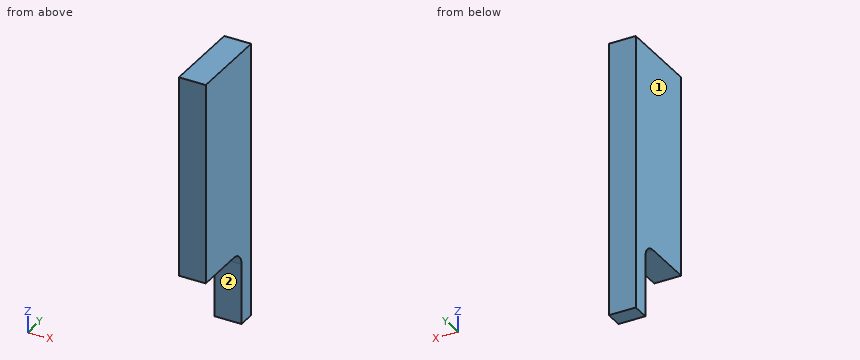
```python
from build123d import *

# Parameters (mm, degrees)
BOSS_EXTRUDE1_DEPTH = 12.7


with BuildPart() as part:
    # Sketch2 → Boss-Extrude1 (new, symmetric)
    with BuildSketch(Plane(origin=(0, 0, 0), x_dir=(0, 0, -1), z_dir=(1, 0, 0))):
        with BuildLine():
            Line((-130, 38.1), (130, 38.1))
            Line((130, 38.1), (130, 21.9))
            Line((130, 21.9), (72.7, 21.9))
            ThreePointArc((72.7, 21.9), (63.719743879, 18.180256121), (60, 9.2))
            Line((60, 9.2), (60, -38.1))
            Line((60, -38.1), (-130, -38.1))
            Line((-130, -38.1), (-130, 38.1))
        make_face()
    extrude(amount=BOSS_EXTRUDE1_DEPTH, both=True)


solid = part.part
```
Input: part model. Units: mm. Frame: model coordinates. Face numbers are marked on the shaded views. A direction names the side the tool comes from. Round coordinates to 2 decimals unless told otherwise and drop trailing zeros. Loops run counter-clockwise (first coordinate to the right, second up) from the corner with the lowest first, then second, coordinate; pieces in that order, holes last.
1) Section query A-A on x = -8.5. Return the cut outline in (y, z), plus the area to 3 significant figures.
Ans:
outline: (-38.1, -60) - (9.2, -60) arc R12.7 cw to (21.9, -72.7) - (21.9, -130) - (38.1, -130) - (38.1, 130) - (-38.1, 130) - close
area: 15,600 mm2
2) Pin query (flat end, axial travel): pin 1 (12.5 mm diameter, centred on x = 2, z = -104.5, fed in from -Y); pin 2 (1.5 mm diameter, centred on x = -7, y = 6, fed in from -Z). Return the tip coordinate at first contact, or that it passes through.
Ans:
pin 1: stops at y = 21.9
pin 2: stops at z = -60
3) Section query C-C on y = 17. Return the cut outline in (x, z), plus the area to 3 significant figures.
Ans:
outline: (-12.7, -62.68) - (12.7, -62.68) - (12.7, 130) - (-12.7, 130) - close
area: 4,890 mm2
4) Material intervals for line 1 (Z direction, x = 8, y = -25); line 2 (Y direction, x = 1.5, z = -93.5); line 3 (Z direction, x = 3.5, y = 19), sorted ascending.
Ans:
line 1: z = -60 to 130
line 2: y = 21.9 to 38.1
line 3: z = -64.62 to 130
5) Set-up query: the marked faces 1 and 2. Return all of +Z, -Z, +X, -X, +Y, -Y with unobstructed straight access to the full face (end or side cutting, diameter ignored); none if empty.
Ans:
face 1: +Z, -Z, -X, +Y, -Y
face 2: -Z, +X, -X, -Y
6) Section query B-B on y = 2.5. Return the cut outline in (x, z).
Ans:
outline: (-12.7, -60) - (12.7, -60) - (12.7, 130) - (-12.7, 130) - close
